Geometry: see drawing. Coordinates: mm, zero at the bounding-box minimum. Coordinates: 2 decimals unless noted, no trailing zeros. Order: outer loops, then holes, each group sorted by start corner. A loop starts at its lowest first (then second) coordinate and runs counter-clockwise, first axis right, second up. Notation, with made-up numbers: M 55.5,10.5 L 85.5,10.5 A30 ccw 85.5,44.5 Z; hole C -1,-25 d7. An arc over 180 degrees is marked long. Answer in a Markdown table with one row per item.
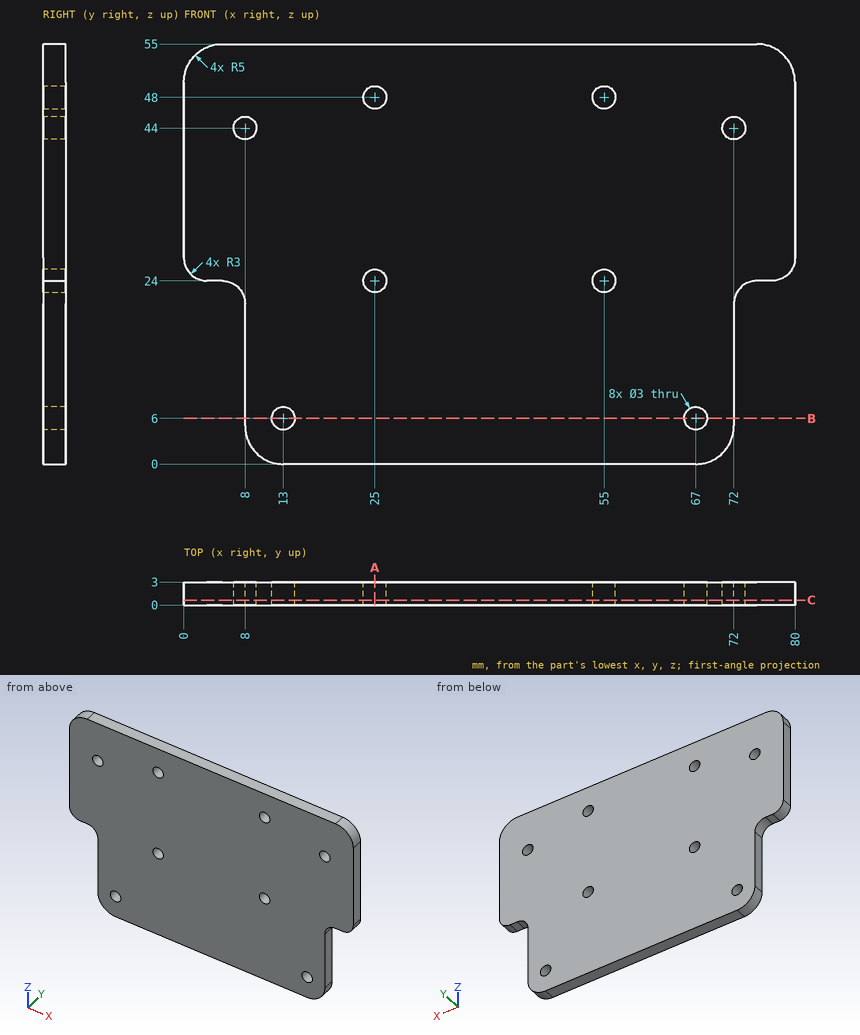
1) Contact query for flat-ended pins moving along their axis: pin 1 (2.5 mm diameter, centred on x = 67, z = 6, fed in from -Y); pin 2 (1 mm diameter, centred on x = 3.5, y = 1.5, fed in from -Z); pin 3 (1 mm diameter, centred on y = 2, z = 26, fed in from +X); pin 4 (1 mm diameter, centred on x = 13, z = 28.5, fed in from -Y). Output: stop coordinate, or through.
Resolved:
| item | result |
|---|---|
| pin 1 | passes through |
| pin 2 | stops at z = 24 |
| pin 3 | stops at x = 79.96 |
| pin 4 | stops at y = 0 |
2) Material intervals for probe 1 along X at (y, z) = (2, 6); probe 2 along X at (y, z) = (1.1, 44); probe 3 along Z at (x, y) = (26, 2.25), sorted ascending.
Resolved:
| item | result |
|---|---|
| probe 1 | x = 8 to 11.5, 14.5 to 65.5, 68.5 to 72 |
| probe 2 | x = 0 to 6.5, 9.5 to 70.5, 73.5 to 80 |
| probe 3 | z = 0 to 22.88, 25.12 to 46.88, 49.12 to 55 |
3) Cut plane C-C, the plane y = 0.65. State how many separate pieces and enclosed holes the cut face has, and give its area (3 significant figures).
Resolved:
| item | result |
|---|---|
| separate pieces | 1 |
| enclosed holes | 8 |
| area | 3,940 mm2 |
4) Cut plane B-B, the plane z = 6. Output: boundary loops of the cut face in (x, y), and give its area (3 significant figures).
Resolved:
| item | result |
|---|---|
| outline | M 8,0 L 11.5,0 L 11.5,3 L 8,3 Z; M 14.5,0 L 65.5,0 L 65.5,3 L 14.5,3 Z; M 68.5,0 L 72,0 L 72,3 L 68.5,3 Z |
| area | 174 mm2 |
5) Cut plane A-A, the plane x = 25. Output: boundary loops of the cut face in (y, z).
Resolved:
| item | result |
|---|---|
| outline | M 0,0 L 3,0 L 3,22.5 L 0,22.5 Z; M 0,25.5 L 3,25.5 L 3,46.5 L 0,46.5 Z; M 0,49.5 L 3,49.5 L 3,55 L 0,55 Z |
